Design review of the part built by this model. Coordinates are the model's own, in mm. A direction names the side the tool comes from. Coordinates: 2 decimals unless noted, no trailing zeros. Order: outer loops, then holes, each group sorted by start corner. A loop starts at its lowest first (then second) coordinate and runs counter-clockwise, first axis right, second up. Notation, with made-up numbers: (51.5, 29) -> (98.5, 29) arc R6 cw to (98.5, 34) -> close; hole circle Ø2 at (71.5, 14.25). An arc over 180 degrees is marked (long way). Write item = value, one per line.
```python
from build123d import *

# Parameters (mm, degrees)
F1_DEPTH = 40


# Not quite as in the source:
# - a feature names something its author has since deleted; it is built from what else it names


with BuildPart() as f1:
    # F0 (on Front) → F1 (new body)
    with BuildSketch(Plane.XZ):
        Polygon((23, 72), (8, 72), (8, 39.8151502013), (8, 36), (23, 36), align=None)
        Polygon((0, 80), (0, 0), (81, 0), (81, 8), (56, 8), (31, 8), (31, 32), (23, 32), (23, 8), (8, 8), (8, 36), (8, 39.8151502013), (8, 72), (8, 80), align=None)
    extrude(amount=-F1_DEPTH)


solid = f1.part
```
(1) We need section B-B (z = 73.5). Write out the cut boundary in (x, y), and give its area (3 significant figures).
Report:
outline = (0, 0) -> (8, 0) -> (8, 40) -> (0, 40) -> close
area = 320 mm²
(2) For L1, parallel to X at y = 25.5, z = 18.5; L2, parallel to Z at x = 15, y = 15.5; L3, parallel to X at y = 16, z = 55.5, list the stretches that pass through material, from the lowest coordinate up.
Report:
L1 = 0 to 8, 23 to 31
L2 = 0 to 8, 36 to 72
L3 = 0 to 23
(3) The part is to be moulded in two halves that separate along X. For faces 6 (the flat face through (16, 20, 8)), 7 (the flat face through (8, 20, 76)), 8 (the flat face through (23, 20, 20)), 9 (the flat face through (25, 40, 31)), say which applies: released by +X, released by -X, zero draft, split by the parting line, or undercut.
Report:
face_6 = undercut
face_7 = released by +X
face_8 = undercut
face_9 = zero draft
(4) We need section C-C (x = 59). Write out the cut boundary in (y, z).
Report:
outline = (0, 0) -> (40, 0) -> (40, 8) -> (0, 8) -> close
(5) For faces 1 (the flat face through (25, 0, 31)), 2 (the flat face through (8, 20, 22)), 3 (the flat face through (27, 20, 32)), 4 (the flat face through (0, 20, 41)), 5 (the flat face through (15, 20, 36)), list the 3-axis set-ups (+Z, -Z, +X, -X, +Y, -Y) from which the entire face can be reached by the end or side of a thin tool; tool diameter is ignored.
Report:
face_1 = +Z, -Z, +X, -X, -Y
face_2 = +Y, -Y
face_3 = +Z, +X, +Y, -Y
face_4 = +Z, -Z, -X, +Y, -Y
face_5 = +X, +Y, -Y
(6) We need section A-A (y = 36). Write out the cut boundary in (x, z).
Report:
outline = (0, 0) -> (81, 0) -> (81, 8) -> (31, 8) -> (31, 32) -> (23, 32) -> (23, 8) -> (8, 8) -> (8, 36) -> (23, 36) -> (23, 72) -> (8, 72) -> (8, 80) -> (0, 80) -> close
(7) Insertion check: pin 1 (6.5 mm diameter, centred on x = 29, y = 15, fed in from +Z); pin 2 (4.5 mm diameter, centred on x = 17.5, y = 28, fed in from +Z); pin 3 (9 mm diameter, centred on y = 15, z = 76, fed in from +X). Each pin has a flat end and moves straight along its axis. Give the tip position at first contact, or say it passes through.
Report:
pin_1 = 32
pin_2 = 72
pin_3 = 23
